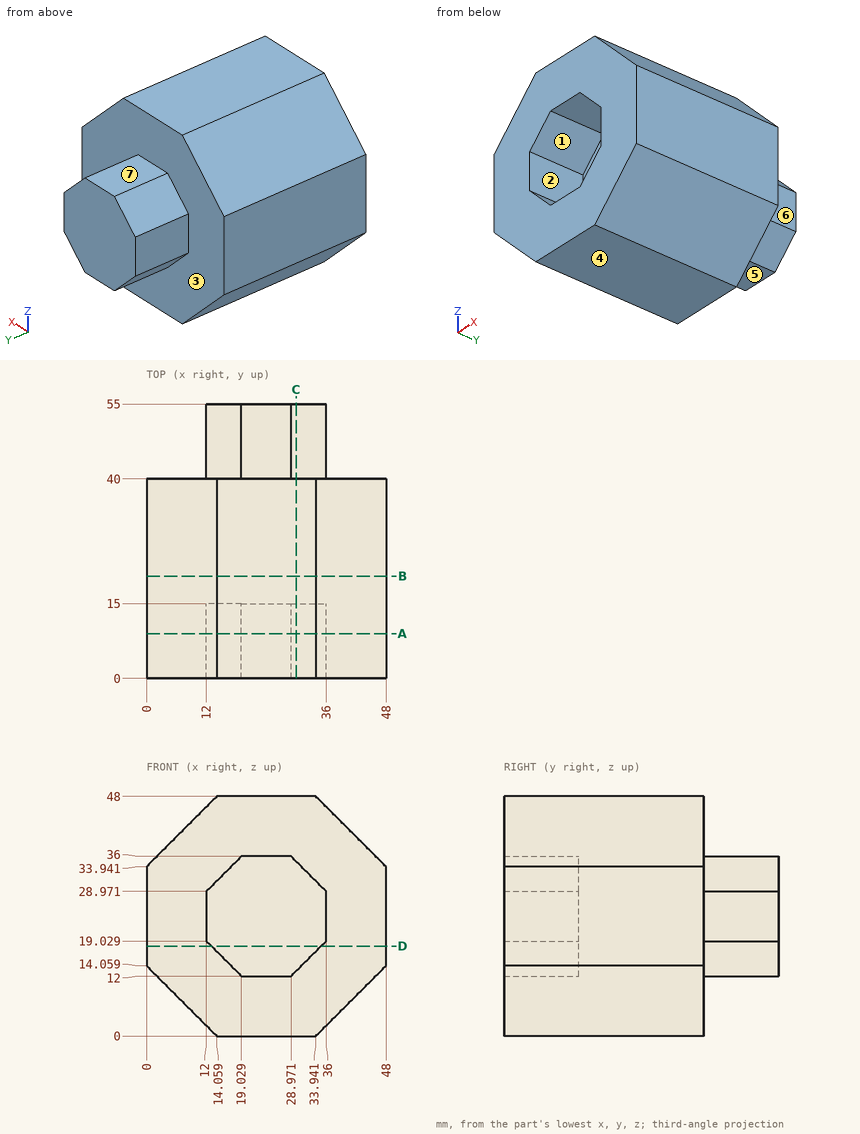
Geometry check sheet. Reference: drawing and pictorial views, mm from the part's lowest x, y, z. A direction names the side the tool comes from. Give positions to 0.01 mm unless a question says otherwise; leave off trailing zeros. Order: outer loops, then holes, each group sorted by start corner. A loop starts at its lowest first (then second) coordinate and runs counter-clockwise, first axis right, second up. Notation, with made-up numbers: M -6,16.25 L 50,16.25 A20 cw 50,22.25 Z; hole C 54.25,29.25 d11. An arc over 180 degrees is marked long. Answer in a Markdown table with one row per item. Add a question column.
Item 1: Mould release check, pull along Z, two halves, no side actions. Record for the marked faces 1, 2, 3 and 4: released by +Z, released by -Z, zero draft, split by the parting line, or undercut.
Item 2: Section check B-B, the plane y = 20.5. Enter the section's corners in (x, z), and give its area (3 significant figures).
Item 3: Tool access check on the marked faces 5, 6 and 7. Record the directions out of +Z, -Z, +X, -X, +Y, -Y that give a thin tool (end or side, any length) a straight path to the whole face; none if there is none.
Item 4: Scan lines: probe 1 along Z at (x, y) = (29, 5.5); probe 2 along Y at (x, z) = (22.5, 42.5); probe 3 along X at (y, z) = (11.5, 16). Record each from-to range of solid material in increasing order. Write a range as from..to.
Item 5: Section check C-C, the plane x = 30. Enter the section's corners in (y, z), and give its area (3 significant figures).
Item 6: Gauge pin test, flat ends, axial feed: pin 1 (3 mm diameter, centred on y = 44.5, z = 24.5, fed in from -X); pin 2 (3 mm diameter, centred on x = 22, y = 44.5, fed in from +Z); pin 3 (7 mm diameter, centred on x = 21.5, z = 22, fed in from -Y); pin 4 (3 mm diameter, centred on y = 46.5, z = 39, fed in from -X). Record the tip position at first contact, or that the pin passes through.
Item 7: Section check A-A, the plane y = 9. Enter the section's corners in (x, z).
Item 8: Section check D-D, the plane z = 18. Enter the section's corners in (x, y), and give its area (3 significant figures).
Filled sheet:
| question | item | result |
|---|---|---|
| 1 | face 1 | undercut |
| 1 | face 2 | undercut |
| 1 | face 3 | zero draft |
| 1 | face 4 | released by -Z |
| 2 | outline | M 0,14.06 L 14.06,0 L 33.94,0 L 48,14.06 L 48,33.94 L 33.94,48 L 14.06,48 L 0,33.94 Z |
| 2 | area | 1,910 mm^2 |
| 3 | face 5 | -Z, +X, -X, +Y |
| 3 | face 6 | +Z, -Z, +X, +Y |
| 3 | face 7 | +Z, +X, -X, +Y |
| 4 | probe 1 | z = 0..12.03, 35.97..48 |
| 4 | probe 2 | y = 0..40 |
| 4 | probe 3 | x = 0..15.03, 32.97..48 |
| 5 | outline | M 0,0 L 40,0 L 40,13.03 L 55,13.03 L 55,34.97 L 40,34.97 L 40,48 L 0,48 L 0,34.97 L 15,34.97 L 15,13.03 L 0,13.03 Z |
| 5 | area | 1,920 mm^2 |
| 6 | pin 1 | stops at x = 12 |
| 6 | pin 2 | stops at z = 36 |
| 6 | pin 3 | stops at y = 15 |
| 6 | pin 4 | passes through |
| 7 | outline | M 0,14.06 L 14.06,0 L 33.94,0 L 48,14.06 L 48,33.94 L 33.94,48 L 14.06,48 L 0,33.94 Z; hole M 12,19.03 L 19.03,12 L 28.97,12 L 36,19.03 L 36,28.97 L 28.97,36 L 19.03,36 L 12,28.97 Z |
| 8 | outline | M 0,0 L 13.03,0 L 13.03,15 L 34.97,15 L 34.97,0 L 48,0 L 48,40 L 34.97,40 L 34.97,55 L 13.03,55 L 13.03,40 L 0,40 Z |
| 8 | area | 1,920 mm^2 |
